Source: CAD feature listing. Evaluate the final solid. Frame: model axes, mm. A direction names the side the tool comes from. Coordinates: 2 decimals unless noted, no trailing zeros. Order: outer loops, then holes, each group sorted by start corner. A loop starts at its lowest first (then second) coordinate and runs counter-clockwise, first axis right, second up.
```python
from build123d import *

# Parameters (mm, degrees)
SKETCH_2_R           = 47.5
SKETCH_2_R_2         = 4
EXTRUDE_1_DEPTH      = 12
SKETCH_3_R           = 45
SKETCH_3_R_2         = 4
EXTRUDE_2_DEPTH      = 1
EXTRUDE_2_DEPTH_BACK = 13
SKETCH_4_R           = 9
SKETCH_4_R_2         = 4
EXTRUDE_3_DEPTH      = 5.2


with BuildPart() as part:
    # 草图2 → 凸台-拉伸1 (new body)
    with BuildSketch(Plane(origin=(0, 0, 0), x_dir=(0, 0, -1), z_dir=(1, 0, 0))):
        Circle(SKETCH_2_R)
        Circle(SKETCH_2_R_2, mode=Mode.SUBTRACT)
    extrude(amount=EXTRUDE_1_DEPTH)

    # 草图3 → 凸台-拉伸2 (add, two sides)
    with BuildSketch(Plane(origin=(12, 0, 0), x_dir=(0, 0, -1), z_dir=(1, 0, 0))) as extrude_2_sk:
        Circle(SKETCH_3_R)
        Circle(SKETCH_3_R_2, mode=Mode.SUBTRACT)
    extrude(amount=EXTRUDE_2_DEPTH)
    extrude(extrude_2_sk.sketch, amount=-EXTRUDE_2_DEPTH_BACK)

    # 草图4 → 凸台-拉伸3 (add)
    with BuildSketch(Plane(origin=(13, 0, 0), x_dir=(0, 0, -1), z_dir=(1, 0, 0))):
        Circle(SKETCH_4_R)
        Circle(SKETCH_4_R_2, mode=Mode.SUBTRACT)
    extrude(amount=EXTRUDE_3_DEPTH)


solid = part.part
```
Q1. Material intervals for line 1 along Y through (x, z) = (17.15, 0); line 2 along Y through (x, z) = (12.6, 0); line 3 along X through (y, z) = (34, 19), sorted ascending.
Solutions:
line 1: y = -9 to -4, 4 to 9
line 2: y = -45 to -4, 4 to 45
line 3: x = -1 to 13
Q2. Set-up query: faces 1 (the cylindrical face through (-0.493, -39.923, -20.765)), 2 (the cylindrical face through (12.493, -39.923, -20.765)), 3 (the flat face through (18.2, -2, -4)). Return all of +Z, -Z, +X, -X, +Y, -Y with unobstructed straight access to the full face (end or side cutting, diameter ignored); none if empty.
Solutions:
face 1: -X
face 2: +X
face 3: +Z, -Z, +X, +Y, -Y
Q3. Section query C-C on x = 15.5. Output: boundary loops of the cut face in (y, z), plus the area to 3 significant figures.
Solutions:
outline: circle Ø18 at (0, 0); hole circle Ø8 at (0, 0)
area: 204 mm2
Q4. Section query D-D on z = -20.5. Output: boundary loops of the cut face in (x, y).
Solutions:
outline: (-1, -40.06) - (0, -40.06) - (0, -42.85) - (12, -42.85) - (12, -40.06) - (13, -40.06) - (13, 40.06) - (12, 40.06) - (12, 42.85) - (0, 42.85) - (0, 40.06) - (-1, 40.06) - close
Q5. Pin query (flat end, axial travel): P1, Ø9, axis at y = 0, z = 0, coming from the -X side; P2, Ø10, axis at x = 6.5, y = -22, coming from the +Z side; P3, Ø1, axis at x = 5.5, y = 7, coming from the +Z side; P4, Ø2, axis at x = 10, y = 21.5, coming from the -Z side. Return the tip coordinate at first contact, or that it passes through.
Solutions:
P1: stops at x = -1
P2: stops at z = 44.35
P3: stops at z = 47.05
P4: stops at z = -42.85
Q6. Section query A-A on y = 0. Output: boundary loops of the cut face in (x, z).
Solutions:
outline: (-1, -45) - (0, -45) - (0, -47.5) - (12, -47.5) - (12, -45) - (13, -45) - (13, -9) - (18.2, -9) - (18.2, -4) - (-1, -4) - close; (-1, 4) - (18.2, 4) - (18.2, 9) - (13, 9) - (13, 45) - (12, 45) - (12, 47.5) - (0, 47.5) - (0, 45) - (-1, 45) - close
